```python
from build123d import *

# Parameters (mm, degrees)
PAD_DEPTH       = 5
CHAMFER_SIZE    = 3
CHAMFER001_SIZE = 3
SKETCH001_R     = 4.474248
SKETCH001_R_2   = 6.533879
SKETCH001_R_3   = 3.458444
SKETCH001_R_4   = 3.797006
POCKET_DEPTH    = 5.001


with BuildPart() as part:
    # Sketch → Pad (new body)
    with BuildSketch(Plane.XY):
        Polygon((0, 0), (30, 0), (50, 9.326153), (50, 24.251131), (20, 24.251131), (0, 20), align=None)
    extrude(amount=PAD_DEPTH)

    # Chamfer
    chamfer_edges = [part.edges().sort_by_distance(p)[0] for p in [
        (0, 0, 2.5),
    ]]
    chamfer(chamfer_edges, length=CHAMFER_SIZE)

    # Chamfer001
    chamfer001_edges = [part.edges().sort_by_distance(p)[0] for p in [
        (50, 24.251131, 2.5),
    ]]
    chamfer(chamfer001_edges, length=CHAMFER001_SIZE)

    # Sketch001 (on Face10 of Chamfer001) → Pocket (cut, through all)
    with BuildSketch(Plane.XY.offset(5)):
        with Locations((13.710362, 14.266204)):
            Circle(SKETCH001_R)
        with Locations((33.767467, 14.130686)):
            Circle(SKETCH001_R_2)
        with Locations((22.451464, 6.473749)):
            Circle(SKETCH001_R_3)
        with Locations((7.002075, 6.202708)):
            Circle(SKETCH001_R_4)
    extrude(amount=-POCKET_DEPTH, mode=Mode.SUBTRACT)


solid = part.part
```
Geometry check sheet. Reference: the model listing, model coordinates, mm. Give positions to 0.01 mm unless a question says otherwise; leave off trailing zeros. Write each loop counter-clockwise with the first axis right and the second up, starting at its lowest first coordinate (ties: lowest second). Pieces come first, ordered by that corner, then holes.
1) Section check D-D, the plane z = 2.65. Record the boundary of the cut face in (x, y), and give its area (3 significant figures).
2) Release check for a two-part mould opening along X. For faces 1 (the flat face through (0, 12, 2)), 2 (the cylindrical face through (28.952, 18.547, 2.535)), 3 (the flat face through (50, 15, 2)) record: pulls with the +X half, pulls with the -X half, needs draft (parallel to the pull), parting line crosses it, or undercut.
3) Material ranges on L1, parallel to X at y = 6.5, z = 2.9; L2, parallel to X at y = 7.25, z = 4.6; L3, parallel to Y at x = 30, z = 4, recorded low to high.
4) Section check A-A, the plane x = 29. Record the boundary of the cut face in (y, z).
5) Gauge pin test, flat ends, axial feed: pin 1 (1 mm diameter, centred on y = 6, z = 3.5, fed in from +X); pin 2 (1 mm diameter, centred on x = 41, y = 3, fed in from -Z); pin 3 (3 mm diameter, centred on x = 6, z = 3, fed in from +Y). Record the tip position at first contact, or that the pin passes through.
6) Section check B-B, the plane y = 19.5. Record the boundary of the cut face in (x, z), and give its area (3 significant figures).
7) Section check C-C, the plane y = 13. Record the boundary of the cut face in (x, z), and give its area (3 significant figures).
Computed:
1. outline: (0, 3) - (3, 0) - (30, 0) - (50, 9.33) - (50, 21.25) - (47, 24.25) - (20, 24.25) - (0, 20) - close; hole circle Ø7.59 at (7, 6.2); hole circle Ø8.95 at (13.71, 14.27); hole circle Ø6.92 at (22.45, 6.47); hole circle Ø13.07 at (33.77, 14.13)
1. area: 788 mm2
2. face 1: pulls with the -X half
2. face 2: undercut
2. face 3: pulls with the +X half
3. L1: x = 0 to 3.22, 10.79 to 18.99, 25.91 to 43.94
3. L2: x = 0 to 3.35, 10.65 to 19.08, 25.82 to 45.55
3. L3: y = 0 to 8.79, 19.47 to 24.25
4. outline: (0, 0) - (9.66, 0) - (9.66, 5) - (0, 5) - close; (18.6, 0) - (24.25, 0) - (24.25, 5) - (18.6, 5) - close
5. pin 1: stops at x = 43.94
5. pin 2: passes through
5. pin 3: stops at y = 21.59
6. outline: (0, 0) - (30.04, 0) - (30.04, 5) - (0, 5) - close; (37.49, 0) - (50, 0) - (50, 5) - (37.49, 5) - close
6. area: 213 mm2
7. outline: (0, 0) - (9.42, 0) - (9.42, 5) - (0, 5) - close; (18, 0) - (27.33, 0) - (27.33, 5) - (18, 5) - close; (40.2, 0) - (50, 0) - (50, 5) - (40.2, 5) - close
7. area: 143 mm2
